from build123d import *

# Parameters (mm, degrees)
FILLET_1_R = 0.5


with BuildPart() as part:
    # 草图1 → 旋转2 (revolve)
    with BuildSketch(Plane.XY):
        with BuildLine():
            Line((1.9, 0.5), (11.9, 0.5))
            Line((11.9, 0.5), (11.9, 0))
            Line((11.9, 0), (4, 0))
            Line((4, 0), (3.266776521, 0))
            Line((3.266776521, 0), (1.729753624, 0))
            Line((1.729753624, 0), (1.2, 0))
            ThreePointArc((1.2, 0), (1.172400412, 0.255885273), (1.090871211, 0.5))
            ThreePointArc((1.090871211, 0.5), (0.887385904, 0.807803353), (0.6, 1.039230485))
            Line((0.6, 1.039230485), (0.982344135, 1.701469953))
            ThreePointArc((0.982344135, 1.701469953), (1.561364608, 1.192535349), (1.9, 0.5))
        make_face()
    revolve(axis=Axis((0, 0, 0), (1, 0, 0)))

    # 圆角1
    fillet_1_edges = [part.edges().sort_by_distance(p)[0] for p in [
        (11.9, -0.5, 0),
        (0.982344135, -1.701469953, 0),
    ]]
    fillet(fillet_1_edges, radius=FILLET_1_R)


solid = part.part
Work out the finished part from the listing and answer in its coordinate system (mm). Give positions to 0.01 mm unless a question says otherwise; leave off trailing zeros. Write each loop counter-clockwise with the first axis right and the second up, starting at its lowest first coordinate (ties: lowest second). Pieces come first, ordered by that corner, then holes.
Q1. Straight lines are drawn through the part: L1, parallel to Z at x = 3.25, y = 0; L2, parallel to X at y = 0.7, z = 0.5; L3, parallel to X at y = -0.25, z = -0.75. For each, find the intervals that lie inside material, in ascending order.
Answer:
L1: z = -0.5 to 0.5
L2: x = 0.84 to 1.77
L3: x = 0.9 to 1.8
Q2. The part is cut by section A-A on x = 4.75. Give the vertices of the cut face in (y, z).
Answer:
outline: circle Ø1 at (0, 0)
Q3. Given pin 1 (1.5 mm diameter, centred on x = 4.5, z = -1, fed in from -Y), flat-ended and moving along its own axis, determine where the tip first touches the part or whether it passes through.
Answer:
pin 1: stops at y = -0.43
